For this review, take the finished solid that the model builds, in its own axes (mm). Face numbers are marked on the shaded views. A direction names the side the tool comes from. Coordinates: 2 decimals unless noted, no trailing zeros. Write each loop counter-clockwise with the first axis right and the second up, starting at its lowest first coordinate (ties: lowest second). Pieces come first, ordered by that corner, then holes.
1) We need section A-A on x = 7. Write out the cut boundary in (y, z).
2) We need section C-C on x = 16. Write out the cut boundary in (y, z).
3) Mouldability with a two-part tool opening along X and no side actions: class the marked faces 1, 2, 3 and 4 as pulls with the +X half, pulls with the -X half, needs draft (parallel to the pull), parting line crosses it, or undercut.
4) To check wall thickness, follow line 1 along X through (y, z) = (2.25, -19.5); line 2 along Z through (x, y) = (13, 10.5); line 3 along Z through (x, y) = (-11.5, 17). State the ranges of each line that lie inside material, in increasing order.
5) We need section B-B on x = -5.5. Write out the cut boundary in (y, z), then the cut area to 3 significant figures.
6) Insertion check: P1, Ø4, axis at y = 15, z = -12.5, coming from the +X side; P2, Ø6, axis at x = -4.5, y = 2.5, coming from the -Z side; P3, Ø9, axis at x = 19, y = 12.5, coming from the +Z side; P4, Ø6, axis at y = 11, z = -1.5, coming from the -X side. Each pin has a flat end and moves straight along its axis. Give the tip position at first contact, or say it passes through.
7) For the marked faces 5, 6, 7 and 8, list the 3-axis set-ups (+Z, -Z, +X, -X, +Y, -Y) from which the entire face can be reached by the end or side of a thin tool; tool diameter is ignored.
from build123d import *
from build123d.topology import SkipClean

# Parameters (mm, degrees)
SKETCH1_W            = 14
SKETCH1_H            = 42
BOSS_EXTRUDE1_DEPTH  = 22.5
FILLET1_R            = 2
BOSS_EXTRUDE2_DEPTH  = 18.5
BOSS_EXTRUDE3_DEPTH  = 5
SKETCH4_R            = 1.1
CUT_EXTRUDE1_DEPTH   = 15
SKETCH5_W            = 2
SKETCH5_H            = 4
BOSS_EXTRUDE4_DEPTH  = 5
BOSS_EXTRUDE5_DEPTH  = 4
CUT_EXTRUDE2_START   = -2
CUT_EXTRUDE2_DEPTH   = 2
SKETCH12_R           = 3.5
SKETCH12_R_2         = 3.070336519
BOSS_EXTRUDE6_DEPTH  = 1
SKETCH14_R           = 3
BOSS_EXTRUDE7_DEPTH  = 1
SKETCH15_R           = 1
BOSS_EXTRUDE8_DEPTH  = 7
SKETCH16_R           = 2
BOSS_EXTRUDE9_DEPTH  = 1.5
CUT_EXTRUDE3_DEPTH   = 18.5
BOSS_EXTRUDE10_START = 32.5
BOSS_EXTRUDE10_DEPTH = 32.5
FILLET2_R            = 3
FILLET3_R            = 3
BOSS_EXTRUDE11_DEPTH = 2
BOSS_EXTRUDE12_DEPTH = 2.2
FILLET4_R            = 1


with BuildPart() as part:
    # Sketch1 → Boss-Extrude1 (new body)
    with BuildSketch(Plane(origin=(0, 0, 0), x_dir=(1, 0, 0), z_dir=(0, 1, 0))):
        with Locations((-14.72963025, -0.456790856)):
            Rectangle(SKETCH1_W, SKETCH1_H)
    extrude(amount=BOSS_EXTRUDE1_DEPTH)

    # Fillet1
    fillet1_edges = [part.edges().sort_by_distance(p)[0] for p in [
        (-14.72963025, 22.5, -20.543209144),
        (-14.72963025, 0, -20.543209144),
        (-14.72963025, 0, 21.456790856),
        (-14.72963025, 22.5, 21.456790856),
    ]]
    fillet(fillet1_edges, radius=FILLET1_R)

    # Sketch2 → Boss-Extrude2 (add)
    with BuildSketch(Plane(origin=(-7.72963025, 0, 0), x_dir=(0, 0, -1), z_dir=(1, 0, 0))):
        with BuildLine():
            Line((3.666133326, 18.67433994), (3.666133326, 3.82566006))
            ThreePointArc((3.666133326, 3.82566006), (12.136760187, 0.056811401), (20.543209144, 3.966716207))
            Line((20.543209144, 3.966716207), (20.543209144, 18.533283793))
            ThreePointArc((20.543209144, 18.533283793), (12.136760187, 22.443188599), (3.666133326, 18.67433994))
        make_face()
    extrude(amount=BOSS_EXTRUDE2_DEPTH)

    # Sketch3 → Boss-Extrude3 (add)
    with BuildSketch(Plane(origin=(-7.72963025, 0, 0), x_dir=(0, 0, -1), z_dir=(1, 0, 0))):
        with BuildLine():
            Line((3.666133326, 12.265446457), (3.666133326, 10.341158941))
            ThreePointArc((3.666133326, 10.341158941), (3.170141933, 10.546427574), (2.72390333, 10.248075799))
            ThreePointArc((2.72390333, 10.248075799), (-1.152649836, 11.204898318), (2.678489822, 12.329861741))
            ThreePointArc((2.678489822, 12.329861741), (3.155102255, 12.033793242), (3.666133326, 12.265446457))
        make_face()
    extrude(amount=BOSS_EXTRUDE3_DEPTH)

    # Sketch4 → Cut-Extrude1 (cut)
    with BuildSketch(Plane(origin=(-7.72963025, 0, 0), x_dir=(0, 0, -1), z_dir=(1, 0, 0))):
        with Locations((-18.956790856, 20)):
            Circle(SKETCH4_R)
        with Locations((-18.956790856, 2.5)):
            Circle(SKETCH4_R)
    extrude(amount=-CUT_EXTRUDE1_DEPTH, mode=Mode.SUBTRACT)

    # Sketch5 → Boss-Extrude4 (add)
    with BuildSketch(Plane(origin=(0, 0, -20.543209144), x_dir=(-1, 0, 0), z_dir=(0, 0, -1))):
        with Locations((7.72963025, 11.25)):
            Rectangle(SKETCH5_W, SKETCH5_H)
    extrude(amount=BOSS_EXTRUDE4_DEPTH)

    # Sketch6 → Boss-Extrude5 (add)
    with BuildSketch(Plane(origin=(-6.72963025, 0, 0), x_dir=(0, 0, -1), z_dir=(1, 0, 0))):
        with BuildLine():
            ThreePointArc((21.679339079, 11.975250565), (21.032871281, 11.616126027), (20.543209144, 12.17031195))
            Line((20.543209144, 12.17031195), (20.543209144, 10.774749435))
            ThreePointArc((20.543209144, 10.774749435), (21.198638933, 11.046780591), (21.679339079, 10.524749435))
            ThreePointArc((21.679339079, 10.524749435), (25.543209144, 11.25), (21.679339079, 11.975250565))
        make_face()
    extrude(amount=BOSS_EXTRUDE5_DEPTH)

    # Sketch7 → Cut-Extrude2 (cut)
    with BuildSketch(Plane(origin=(-6.72963025, 0, 0), x_dir=(0, 0, -1), z_dir=(1, 0, 0)).offset(CUT_EXTRUDE2_START)):
        with BuildLine():
            Line((23.543209144, 13.25), (23.543209144, 13.967200788))
            Line((23.543209144, 13.967200788), (25.760178749, 13.967200788))
            Line((25.760178749, 13.967200788), (25.760178749, 8.970470958))
            Line((25.760178749, 8.970470958), (23.543209144, 8.970470958))
            Line((23.543209144, 8.970470958), (23.543209144, 9.25))
            ThreePointArc((23.543209144, 9.25), (25.543209144, 11.25), (23.543209144, 13.25))
        make_face()
    extrude(amount=CUT_EXTRUDE2_DEPTH, mode=Mode.SUBTRACT)

    # Sketch12 → Boss-Extrude6 (add)
    with BuildSketch(Plane.ZY.offset(21.72963025)):
        with Locations(Location((10.456790856, 11.25, 0), (0, 0, 180))):
            Circle(SKETCH12_R)
        with Locations((10.456790856, 11.25)):
            Circle(SKETCH12_R_2, mode=Mode.SUBTRACT)
    extrude(amount=BOSS_EXTRUDE6_DEPTH)

    # Sketch14 → Boss-Extrude7 (add)
    with BuildSketch(Plane.ZY.offset(21.72963025)):
        with Locations(Location((10.456790856, 11.25, 0), (0, 0, 180))):
            Circle(SKETCH14_R)
    extrude(amount=BOSS_EXTRUDE7_DEPTH)

    # Sketch15 → Boss-Extrude8 (add)
    with SkipClean():  # the faces are left unmerged after this step: merging them gives an invalid solid
        with BuildSketch(Plane.ZY.offset(22.72963025)):
            with BuildLine():
                Line((8.853884636, 8.714119157), (8.853884636, 13.785880843))
                ThreePointArc((8.853884636, 13.785880843), (10.456790856, 14.25), (12.059697077, 13.785880843))
                Line((12.059697077, 13.785880843), (12.059697077, 8.714119157))
                ThreePointArc((12.059697077, 8.714119157), (10.456790856, 8.25), (8.853884636, 8.714119157))
            make_face()
            with Locations((10.456790856, 11.25)):
                Circle(SKETCH15_R, mode=Mode.SUBTRACT)
        extrude(amount=BOSS_EXTRUDE8_DEPTH)

    # Sketch16 → Boss-Extrude9 (add)
    with SkipClean():  # the faces are left unmerged after this step: merging them gives an invalid solid
        with BuildSketch(Plane.ZY.offset(21.72963025)):
            with Locations(Location((-0.543209144, 11.25, 0), (0, 0, 180))):
                Circle(SKETCH16_R)
        extrude(amount=BOSS_EXTRUDE9_DEPTH)

    # Sketch17 → Cut-Extrude3 (cut)
    with SkipClean():  # the faces are left unmerged after this step: merging them gives an invalid solid
        with BuildSketch(Plane(origin=(10.77036975, 0, 0), x_dir=(0, 0, -1), z_dir=(1, 0, 0))):
            with BuildLine():
                Line((19.843209144, 4.230369564), (19.843209144, 18.269630436))
                ThreePointArc((19.843209144, 18.269630436), (12.134214683, 21.743184905), (4.366133326, 18.403860381))
                Line((4.366133326, 18.403860381), (4.366133326, 4.096139619))
                ThreePointArc((4.366133326, 4.096139619), (12.134214683, 0.756815095), (19.843209144, 4.230369564))
            make_face()
        extrude(amount=-CUT_EXTRUDE3_DEPTH, mode=Mode.SUBTRACT)

    # Sketch18 → Boss-Extrude10 (add)
    with SkipClean():  # the faces are left unmerged after this step: merging them gives an invalid solid
        with BuildSketch(Plane(origin=(-7.72963025, 0, 0), x_dir=(0, 0, -1), z_dir=(1, 0, 0)).offset(BOSS_EXTRUDE10_START)):
            with BuildLine():
                Line((19.843209144, 4.230369564), (19.843209144, 18.269630436))
                ThreePointArc((19.843209144, 18.269630436), (12.134214683, 21.743184905), (4.366133326, 18.403860381))
                Line((4.366133326, 18.403860381), (4.366133326, 4.096139619))
                ThreePointArc((4.366133326, 4.096139619), (12.134214683, 0.756815095), (19.843209144, 4.230369564))
            make_face()
        extrude(amount=-BOSS_EXTRUDE10_DEPTH)

    # Fillet2
    # the kernel refuses this fillet: 3 mm, written as the material it takes off along each edge
    with BuildSketch(Plane(origin=(24.77036975, 11.25, -12.043209144), x_dir=(0, -0.03508404520009265, 0.9993843653832083), z_dir=(0, 0.9993843653832083, 0.03508404520009265))) as fillet2_piece_1:
        with BuildLine():
            CenterArc((10.493579535 - FILLET2_R, -FILLET2_R), FILLET2_R, 0, 90)
            Line((10.493579535 - FILLET2_R, 0), (10.493579535, 0))
            Line((10.493579535, 0), (10.493579535, -FILLET2_R))
        make_face()
    revolve(axis=Axis((24.77036975, 11.25, -12.043209144), (1, 0, 0)), revolution_arc=176.972646772, mode=Mode.SUBTRACT)
    with BuildSketch(Plane(origin=(24.77036975, -3.269630436, -19.843209144), x_dir=(-1, 0, 0), z_dir=(0, 1, 0))) as fillet2_piece_2:
        with BuildLine():
            CenterArc((FILLET2_R, FILLET2_R), FILLET2_R, 180, 90)
            Line((0, FILLET2_R), (0, 0))
            Line((0, 0), (FILLET2_R, 0))
        make_face()
    extrude(amount=29.039260873, mode=Mode.SUBTRACT)
    with BuildSketch(Plane(origin=(24.77036975, 11.25, -12.043209144), x_dir=(0, 0.017745103398297987, -0.9998425432563788), z_dir=(0, -0.9998425432563788, -0.017745103398297987))) as fillet2_piece_3:
        with BuildLine():
            CenterArc((10.493579535 - FILLET2_R, -FILLET2_R), FILLET2_R, 0, 90)
            Line((10.493579535 - FILLET2_R, 0), (10.493579535, 0))
            Line((10.493579535, 0), (10.493579535, -FILLET2_R))
        make_face()
    revolve(axis=Axis((24.77036975, 11.25, -12.043209144), (1, 0, 0)), revolution_arc=176.972646772, mode=Mode.SUBTRACT)
    with BuildSketch(Plane(origin=(24.77036975, 25.903860381, -4.366133326), x_dir=(-1, 0, 0), z_dir=(0, -1, 0))) as fillet2_piece_4:
        with BuildLine():
            CenterArc((FILLET2_R, FILLET2_R), FILLET2_R, 180, 90)
            Line((0, FILLET2_R), (0, 0))
            Line((0, 0), (FILLET2_R, 0))
        make_face()
    extrude(amount=29.307720762, mode=Mode.SUBTRACT)

    # Fillet3
    fillet3_edges = [part.edges().sort_by_distance(p)[0] for p in [
        (16.27036975, 4.096139619, -4.366133326),
        (16.27036975, 18.403860381, -4.366133326),
        (16.27036975, 18.269630436, -19.843209144),
        (16.27036975, 4.230369564, -19.843209144),
        (23.939626378, 17.904127425, -18.915484598),
        (23.939626378, 4.595872575, -18.915484598),
        (23.942018914, 18.027736711, -5.296365269),
        (23.942018914, 4.472263289, -5.296365269),
    ]]
    fillet(fillet3_edges, radius=FILLET3_R)

    # Sketch19 → Boss-Extrude11 (add)
    with BuildSketch(Plane(origin=(-2.72963025, 0, 0), x_dir=(0, 0, -1), z_dir=(1, 0, 0))):
        with BuildLine():
            Line((0.768030026, 13.473431353), (0.768030026, 13.968221025))
            Line((0.768030026, 13.968221025), (3.666133326, 13.968221025))
            Line((3.666133326, 13.968221025), (3.666133326, 8.531778975))
            Line((3.666133326, 8.531778975), (0.768030026, 8.531778975))
            Line((0.768030026, 8.531778975), (0.768030026, 9.026568647))
            ThreePointArc((0.768030026, 9.026568647), (-1.590616444, 11.25), (0.768030026, 13.473431353))
        make_face()
        with BuildLine():
            Line((23.505490349, 8.531778975), (23.505490349, 9.026568647))
            ThreePointArc((23.505490349, 9.026568647), (25.864136819, 11.25), (23.505490349, 13.473431353))
            Line((23.505490349, 13.473431353), (23.505490349, 13.968221025))
            Line((23.505490349, 13.968221025), (20.607387049, 13.968221025))
            Line((20.607387049, 13.968221025), (20.607387049, 8.531778975))
            Line((20.607387049, 8.531778975), (23.505490349, 8.531778975))
        make_face()
    extrude(amount=BOSS_EXTRUDE11_DEPTH)

    # Sketch22 → Boss-Extrude12 (add, symmetric)
    with BuildSketch(Plane(origin=(0, 11.25, 0), x_dir=(-1, 0, 0), z_dir=(0, -1, 0))):
        with BuildLine():
            Line((0.72963025, 3.208547986), (0.72963025, 2.217081676))
            Line((0.72963025, 2.217081676), (-10.91025311, 2.217081676))
            Line((-10.91025311, 2.217081676), (-24.765511007, 3.274279543))
            ThreePointArc((-24.765511007, 3.274279543), (-25.380466801, 3.60490992), (-25.6047274, 4.26611659))
            Line((-25.6047274, 4.26611659), (-25.6047274, 19.94322588))
            ThreePointArc((-25.6047274, 19.94322588), (-25.380466801, 20.604432549), (-24.765511007, 20.935062926))
            Line((-24.765511007, 20.935062926), (-10.91025311, 21.992260794))
            Line((-10.91025311, 21.992260794), (0.72963025, 21.992260794))
            Line((0.72963025, 21.992260794), (0.72963025, 21.000794484))
            Line((0.72963025, 21.000794484), (-10.91025311, 21.000794484))
            Line((-10.91025311, 21.000794484), (-24.77036975, 19.94322588))
            Line((-24.77036975, 19.94322588), (-24.77036975, 4.26611659))
            Line((-24.77036975, 4.26611659), (-10.91025311, 3.208547986))
            Line((-10.91025311, 3.208547986), (0.72963025, 3.208547986))
        make_face()
    extrude(amount=BOSS_EXTRUDE12_DEPTH, both=True)

    # Fillet4
    fillet4_edges = [part.edges().sort_by_distance(p)[0] for p in [
        (-0.72963025, 11.25, -21.992260794),
        (-0.72963025, 11.25, -2.217081676),
    ]]
    fillet(fillet4_edges, radius=FILLET4_R)


solid = part.part
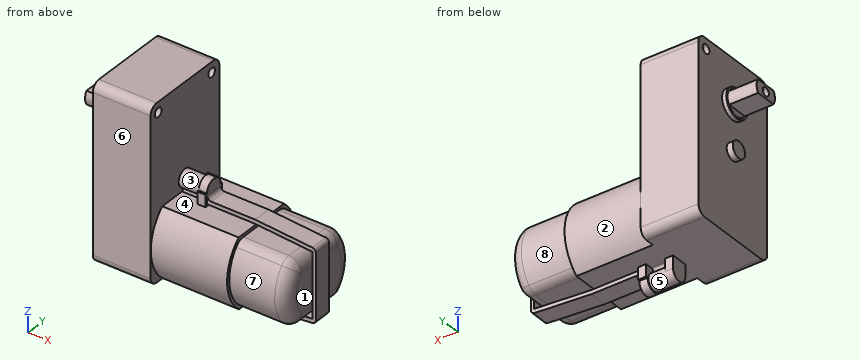
Result:
1. outline: (3.83, -3.67) arc R11.19 ccw to (3.97, -20.54) - (18.53, -20.54) arc R11.19 ccw to (18.67, -3.67) - close; (9.05, -21.99) - (13.45, -21.99) - (13.45, -21) - (9.05, -21) - close; (9.05, -3.21) - (13.45, -3.21) - (13.45, -2.22) - (9.05, -2.22) - close
2. outline: (3.05, -5.49) arc R10.49 ccw to (3.19, -18.76) arc R3 ccw to (5.5, -19.84) - (17, -19.84) arc R3 ccw to (19.31, -18.76) arc R10.49 ccw to (19.45, -5.49) arc R3 ccw to (17.1, -4.37) - (5.4, -4.37) arc R3 ccw to start; (9.05, -21.6) - (13.45, -21.6) - (13.45, -20.61) - (9.05, -20.61) - close; (9.05, -3.6) - (13.45, -3.6) - (13.45, -2.61) - (9.05, -2.61) - close
3. face 1: pulls with the +X half
3. face 2: needs draft
3. face 3: undercut
3. face 4: undercut
4. line 1: x = -21.73 to -7.73
4. line 2: z = -21.83 to -20.84, -19.84 to -4.37, -3.37 to -2.38
4. line 3: z = -20.54 to 21.46
5. outline: (3.83, -3.67) arc R11.19 ccw to (3.97, -20.54) - (10.77, -20.54) arc R0.62 cw to (10.52, -21.68) arc R2 ccw (long way) to (11.98, -21.68) arc R0.59 cw to (12.17, -20.54) - (18.53, -20.54) arc R11.19 ccw to (18.67, -3.67) - (12.27, -3.67) arc R0.6 cw to (12.33, -2.68) arc R2.07 ccw (long way) to (10.25, -2.72) arc R0.57 cw to (10.34, -3.67) - close
5. area: 366 mm2
6. P1: stops at x = 25.6
6. P2: stops at z = -20.54
6. P3: stops at z = -2.49
6. P4: stops at x = -23.23
7. face 5: none
7. face 6: +Z, -Z, +X, -X, -Y
7. face 7: +X, -Y
7. face 8: +X, +Y
